For this review, take the finished solid that the model builds, in its own axes (mm). A direction names the side the tool comes from. Round coordinates to 2 decimals unless told otherwise and drop trailing zeros. Write each loop counter-clockwise with the first axis right and the second up, starting at its lowest first coordinate (ties: lowest second). Pieces come first, ordered by that corner, then holes.
from build123d import *

# Parameters (mm, degrees)
F1_DEPTH = 133.35
F2_W     = 6.477
F2_H     = 34.5941142
F5_DEPTH = 6.35
F6_R     = 1.778
F7_DEPTH = 25.4


with BuildPart() as f1:
    # F0 (on Front) → F1 (new body)
    with BuildSketch(Plane.XZ):
        Polygon((-23.3606961086, -17.2970571), (23.3606961086, 17.2970571), (23.3606961086, 23.7740571), (-7.9238067593, 0.6099429), (-23.3606961086, 0.6099429), (-28.8964977668, 0.6099429), (-23.3606961086, -10.8200571), (-61.4606961086, -17.2970571), align=None)
    extrude(amount=F1_DEPTH)

    # F2 (on face) → F3 (join, up to the next surface of F1)
    with BuildSketch(Plane.YZ.offset(23.3606961086)):
        with Locations((-130.1115, 0)):
            Rectangle(F2_W, F2_H)
        with Locations((-3.2385, 0)):
            Rectangle(F2_W, F2_H)
    extrude(until=Until.NEXT, dir=(-1, 0, 0))

    # F4 (on face) → F5 (join)
    with BuildSketch(Plane.YZ.offset(23.3606961086)):
        Polygon((0, 23.7740571), (-133.35, 23.7740571), (-133.35, 17.2970571), (-126.873, 17.2970571), (-6.477, 17.2970571), (0, 17.2970571), align=None)
    extrude(amount=F5_DEPTH)

    # F6 (on face) → F7 (cut)
    with BuildSketch(Plane.XY.offset(23.7740571)):
        with Locations((26.5356961086, -38.3286)):
            Circle(F6_R)
        with Locations((26.5356961086, -47.7774)):
            Circle(F6_R)
        with Locations((26.5356961086, -57.2262)):
            Circle(F6_R)
        with Locations((26.5356961086, -66.675)):
            Circle(F6_R)
        with Locations((26.5356961086, -76.1238)):
            Circle(F6_R)
        with Locations((26.5356961086, -85.5726)):
            Circle(F6_R)
        with Locations((26.5356961086, -95.0214)):
            Circle(F6_R)
    extrude(amount=-F7_DEPTH, mode=Mode.SUBTRACT)


solid = f1.part
(1) Mouldability with a two-part tool opening along X and no side actions: class faces 6 (the face through (-42.144, -65.742, -14.013)), 7 (the face through (27.356, -39.906, 20.581)), 8 (the face through (0, -66, 0)) as pulls with the +X half, pulls with the -X half, needs draft (parallel to the pull), parting line crosses it, or undercut.
Geometry check:
face 6: pulls with the -X half
face 7: undercut
face 8: pulls with the +X half
(2) For pin 1 Ø6.5 at (x, y) = (-16, -49) entering from +Z; pin 2 Ø4 at (y, z) = (-99.5, 17) entering from -X; pin 3 Ø2 at (x, y) = (-52.5, -97.5) entering from +Z, all flat-tipped, find the tip position at first contact; note any pin that passes through.
Geometry check:
pin 1: stops at z = 0.61
pin 2: stops at x = 11.51
pin 3: stops at z = -15.6
(3) We need section B-B, the plane x = 3.5. Give the boundary of the cut face in (y, z).
Geometry check:
outline: (-133.35, -17.3) - (-126.87, -17.3) - (-126.87, 2.59) - (-6.48, 2.59) - (-6.48, -17.3) - (0, -17.3) - (0, 9.07) - (-133.35, 9.07) - close
(4) We need section D-D, the plane z = 13.5. Give the boundary of the cut face in (x, y).
Geometry check:
outline: (9.48, -133.35) - (23.36, -133.35) - (23.36, -126.87) - (18.23, -126.87) - (18.23, -6.48) - (23.36, -6.48) - (23.36, 0) - (9.48, 0) - close
(5) For faces 1 (the face through (23.361, -130, 0)), 2 (the face through (1, 0, -4)), 3 (the face through (6, -6.477, -4)), 4 (the face through (-26.167, -65.742, -5.025)), 5 (the face through (27.492, -65.176, 20.581)), list the 3-axis set-ups (+Z, -Z, +X, -X, +Y, -Y) from which the entire face can be reached by the end or side of a thin tool; tool diameter is ignored.
Geometry check:
face 1: -Z, +X, +Y, -Y
face 2: +Z, -Z, +X, -X, +Y
face 3: -Z, +X
face 4: -X, +Y, -Y
face 5: +Z, -Z
(6) For line 1 along Y through (x, z) = (1, -0.5); line 2 along Z through (x, y) = (-23.5, -55); line 3 along X through (y, z) = (-19, 19), list the stretches that pass through material, from the lowest coordinate up.
Geometry check:
line 1: y = -133.35 to -126.87, -6.48 to 0
line 2: z = -17.3 to -10.84, -10.53 to 0.61
line 3: x = 16.91 to 29.71
(7) We need section A-A, the plane y = -42. Give the boundary of the cut face in (x, z), and give its area (3 significant figures).
Geometry check:
outline: (-61.46, -17.3) - (-23.36, -17.3) - (23.36, 17.3) - (29.71, 17.3) - (29.71, 23.77) - (23.36, 23.77) - (-7.92, 0.61) - (-28.9, 0.61) - (-23.36, -10.82) - close
area: 587 mm2
(8) We need section C-C, the plane z = 20.5. Give the boundary of the cut face in (x, y) (3 decimals), and give its area (3 significant figures).
Geometry check:
outline: (18.939, -133.35) - (29.711, -133.35) - (29.711, 0) - (18.939, 0) - close; hole circle Ø3.556 at (26.536, -95.021); hole circle Ø3.556 at (26.536, -85.573); hole circle Ø3.556 at (26.536, -76.124); hole circle Ø3.556 at (26.536, -66.675); hole circle Ø3.556 at (26.536, -57.226); hole circle Ø3.556 at (26.536, -47.777); hole circle Ø3.556 at (26.536, -38.329)
area: 1,370 mm2
